Read the model definition and answer for the solid it produces. Units are mm, in the model's axes. Coordinates: 2 decimals unless noted, no trailing zeros. Write each loop counter-clockwise with the first axis right and the second up, starting at its lowest first coordinate (ties: lowest second). Pieces come first, ordered by that corner, then holes. Notation, with made-up numbers: (24.25, 36.5) -> (74.25, 36.5) arc R16 ccw to (74.25, 58.5) -> close; hole circle Ø7 at (66, -34.5). An arc over 180 degrees is marked (long way). Write item = value, one per line. Start each with the question number.
1) Flat-ended cylindrical pins translate along their axes: pin 1 Ø3 at (x, z) = (5, 2) entering from +Y; pin 2 Ø6 at (x, y) = (-5.5, -5) entering from -Z. Find the tip coordinate at first contact, or state that the pin passes through.
2) For a pull along Y with two mould halves and no side action, classify faces 1 (the face through (0, -15, 2)), 2 (the face through (8.775, -0.199, 2.465)), 3 (the face through (0, -3, 0)) as released by +Y, released by -Y, zero draft, split by the parting line, or undercut.
3) Section A-A (z = 2) is taken. Determine the outline of the cut face in (x, y).
4) Find the intervals of material crossed by line 1 along Y through (x, z) = (6.5, 1.95); line 2 along Y through (x, z) = (-10, 0.45); line 3 along X through (y, z) = (-10.5, 1.4), in increasing order. Write a range as from..to.
5) Section C-C (y = -4.25) is taken. Determine the outline of the cut face in (x, z).
6) Section B-B (x = -9) is taken. Determine the outline of the cut face in (y, z), plus the area to 3 significant figures.
from build123d import *

# Parameters (mm, degrees)
F1_DEPTH = 5
F2_SIZE  = 0.7
F3_R     = 0.4


with BuildPart() as f1:
    # F0 (on Top) → F1 (new body)
    with BuildSketch(Plane.XY):
        Polygon((0, 15), (-17.3205080757, -15), (17.3205080757, -15), align=None)
    extrude(amount=F1_DEPTH)

    # F2
    f2_edges = [f1.edges().sort_by_distance(p)[0] for p in [
        (-17.320508, -15, 2.5),
        (17.320508, -15, 2.5),
        (0, 15, 2.5),
    ]]
    chamfer(f2_edges, length=F2_SIZE)

    # F3
    f3_edges = [f1.edges().sort_by_distance(p)[0] for p in [
        (-0.35, 14.393782, 2.5),
        (0.35, 14.393782, 2.5),
        (16.970508, -14.393782, 2.5),
        (16.620508, -15, 2.5),
        (-16.620508, -15, 2.5),
        (-16.970508, -14.393782, 2.5),
    ]]
    fillet(f3_edges, radius=F3_R)


solid = f1.part
Answer key:
q1.pin_1 = 8.94
q1.pin_2 = 0
q2.face_1 = released by -Y
q2.face_2 = released by +Y
q2.face_3 = zero draft
q3.outline = (-16.86, -14.59) -> (-16.74, -14.8) arc R0.4 ccw to (-16.39, -15) -> (16.39, -15) arc R0.4 ccw to (16.74, -14.8) -> (16.86, -14.59) arc R0.4 ccw to (16.86, -14.19) -> (0.47, 14.19) arc R0.4 ccw to (0.12, 14.39) -> (-0.12, 14.39) arc R0.4 ccw to (-0.47, 14.19) -> (-16.86, -14.19) arc R0.4 ccw to start
q4.line_1 = -15..3.74
q4.line_2 = -15..-2.32
q4.line_3 = -14.72..14.72
q5.outline = (-11.11, 0) -> (11.11, 0) -> (11.11, 5) -> (-11.11, 5) -> close
q6.outline = (-15, 0) -> (-0.59, 0) -> (-0.59, 5) -> (-15, 5) -> close
q6.area = 72.1 mm^2
